Job drawing, mm, ordinate dimensions from the low corner. One solid piece. Round coordinates to 2 decimals unless told otherwise and drop trailing zeros. Write each loop counter-clockwise with the first axis right and the second up, starting at its lowest first coordinate (ties: lowest second). Pieces come first, ordered by that corner, then holes.
1) Wall check: probe 1 along X at (y, z) = (7.25, 2.3); probe 2 along Y at (x, z) = (12.5, 2); probe 3 along X at (y, z) = (7, 1.4). Give the ranges that are in metal, low to high.
2) Flat gauge pin, fed straight in: pin 1 (2 mm diameter, centred on x = 87.5, y = 6, fed in from -Z). Where does the tip first touch, or does it go through?
3) Saw through at D-D (x = 88). Write the cut outline in (y, z).
4) Saw through at B-B (y = 6). Write the cut outline in (x, z).
5) Saw through at C-C (z = 0.75). Write the cut outline in (x, y).
6) Saw through at A-A (x = 37.5). Write the cut outline in (y, z), plus the area to 3 significant figures.
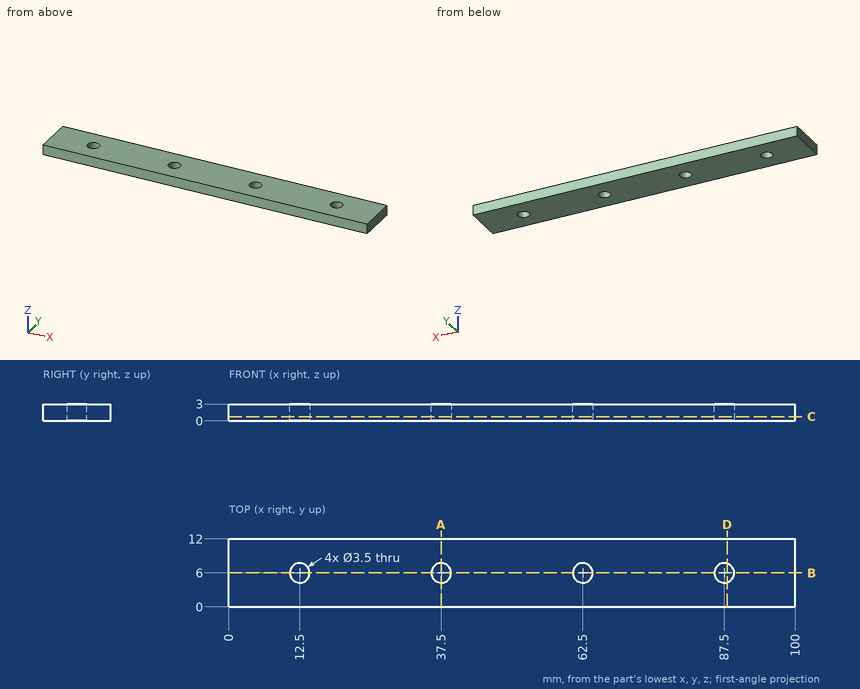
Evaluation:
1. probe 1: x = 0 to 11.28, 13.72 to 36.28, 38.72 to 61.28, 63.72 to 86.28, 88.72 to 100
1. probe 2: y = 0 to 4.25, 7.75 to 12
1. probe 3: x = 0 to 11.06, 13.94 to 36.06, 38.94 to 61.06, 63.94 to 86.06, 88.94 to 100
2. pin 1: passes through
3. outline: (0, 0) - (4.32, 0) - (4.32, 3) - (0, 3) - close; (7.68, 0) - (12, 0) - (12, 3) - (7.68, 3) - close
4. outline: (0, 0) - (10.75, 0) - (10.75, 3) - (0, 3) - close; (14.25, 0) - (35.75, 0) - (35.75, 3) - (14.25, 3) - close; (39.25, 0) - (60.75, 0) - (60.75, 3) - (39.25, 3) - close; (64.25, 0) - (85.75, 0) - (85.75, 3) - (64.25, 3) - close; (89.25, 0) - (100, 0) - (100, 3) - (89.25, 3) - close
5. outline: (0, 0) - (100, 0) - (100, 12) - (0, 12) - close; hole circle Ø3.5 at (12.5, 6); hole circle Ø3.5 at (37.5, 6); hole circle Ø3.5 at (62.5, 6); hole circle Ø3.5 at (87.5, 6)
6. outline: (0, 0) - (4.25, 0) - (4.25, 3) - (0, 3) - close; (7.75, 0) - (12, 0) - (12, 3) - (7.75, 3) - close
6. area: 25.5 mm2
